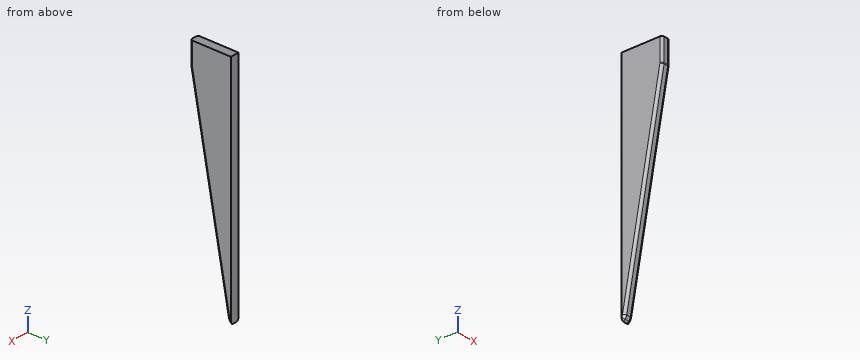
```python
from build123d import *

# Parameters (mm, degrees)
F1_DEPTH     = 19.05
F2_T1_DEPTH  = 453.2334559577
F2_T3_DEPTH  = 17.7217096423
F2_T5_DEPTH  = 62.3469086479
F2_T8_ANGLE  = 10.3758449201
F2_T10_ANGLE = 34.6241550799
F2_T12_ANGLE = 10.3758449201
F2_T14_ANGLE = 34.6241550799


# Not quite as in the source:
# - a fillet or chamfer that OpenCascade refuses, or shapes differently, is made with other operations: its cross-section is extruded or revolved along the edge and cut away or added


with BuildPart() as f1:
    # F0 (on Right) → F1 (new body)
    with BuildSketch(Plane.YZ):
        with BuildLine():
            Line((42.4285726043, -178.7500022879), (42.4285726043, 329.2499977121))
            Line((42.4285726043, 329.2499977121), (-46.4714273957, 329.2499977121))
            Line((-46.4714273957, 329.2499977121), (-46.4714273957, 279.6030890642))
            ThreePointArc((-46.4714273957, 279.6030890642), (-46.4194016068, 278.4547213725), (-46.2637504894, 277.3157623006))
            Line((-46.2637504894, 277.3157623006), (35.3656206904, -168.5061879892))
            ThreePointArc((35.3656206904, -168.5061879892), (36.6122005726, -172.1199848152), (38.877687663, -175.1991173466))
            Line((38.877687663, -175.1991173466), (42.4285726043, -178.7500022879))
        make_face()
    extrude(amount=F1_DEPTH)

    # F2: fillet of radius 5.08 on 2 edges, made by hand

    # F2_s2 → F2_t1 (cut)
    with BuildSketch(Plane(origin=(0, -50.6297547862, 276.5163530631), x_dir=(1, 0, 0), z_dir=(0, 0.1801044696, -0.9836474877))):
        with BuildLine():
            ThreePointArc((13.97, -4.4385863345), (17.5621024484, -5.9264838861), (19.05, -9.5185863345))
            Line((19.05, -9.5185863345), (19.05, -4.4385863345))
            Line((19.05, -4.4385863345), (13.97, -4.4385863345))
        make_face()
        with BuildLine():
            ThreePointArc((5.08, -4.4385863345), (1.4878975516, -5.9264838861), (0, -9.5185863345))
            Line((0, -9.5185863345), (0, -4.4385863345))
            Line((0, -4.4385863345), (5.08, -4.4385863345))
        make_face()
    extrude(amount=F2_T1_DEPTH, mode=Mode.SUBTRACT)

    # F2_s4 → F2_t3 (cut)
    with BuildSketch(Plane(origin=(0, 107.0384025048, -107.0384025048), x_dir=(1, 0, 0), z_dir=(0, 0.7071067812, -0.7071067812))):
        with BuildLine():
            ThreePointArc((5.08, 96.3938073503), (1.4878975516, 94.9059097987), (0, 91.3138073503))
            Line((0, 91.3138073503), (0, 96.3938073503))
            Line((0, 96.3938073503), (5.08, 96.3938073503))
        make_face()
        with BuildLine():
            ThreePointArc((13.97, 96.3938073503), (17.5621024484, 94.9059097987), (19.05, 91.3138073503))
            Line((19.05, 91.3138073503), (19.05, 96.3938073503))
            Line((19.05, 96.3938073503), (13.97, 96.3938073503))
        make_face()
    extrude(amount=F2_T3_DEPTH, mode=Mode.SUBTRACT)

    # F2_s6 → F2_t5 (cut)
    with BuildSketch(Plane.XY.offset(279.6030890642)):
        with BuildLine():
            ThreePointArc((5.08, -46.4714273957), (1.4878975516, -44.9835298442), (0, -41.3914273957))
            Line((0, -41.3914273957), (0, -46.4714273957))
            Line((0, -46.4714273957), (5.08, -46.4714273957))
        make_face()
        with BuildLine():
            ThreePointArc((13.97, -46.4714273957), (17.5621024484, -44.9835298442), (19.05, -41.3914273957))
            Line((19.05, -41.3914273957), (19.05, -46.4714273957))
            Line((19.05, -46.4714273957), (13.97, -46.4714273957))
        make_face()
    extrude(amount=F2_T5_DEPTH, mode=Mode.SUBTRACT)

    # F2_s7 → F2_t8 (revolve, cut)
    with BuildSketch(Plane.XY.offset(279.6030890642)):
        with BuildLine():
            ThreePointArc((5.08, -46.4714273957), (1.4878975516, -44.9835298442), (0, -41.3914273957))
            Line((0, -41.3914273957), (0, -46.4714273957))
            Line((0, -46.4714273957), (5.08, -46.4714273957))
        make_face()
    revolve(axis=Axis((0, -33.7714273957, 279.6030890642), (1, 0, 0)), revolution_arc=F2_T8_ANGLE, mode=Mode.SUBTRACT)

    # F2_s9 → F2_t10 (revolve, cut)
    with BuildSketch(Plane(origin=(0, 30.9996163936, -169.3055972266), x_dir=(1, 0, 0), z_dir=(0, -0.1801044696, 0.9836474877))):
        with BuildLine():
            ThreePointArc((5.08, 4.4385863345), (1.4878975516, 5.9264838861), (0, 9.5185863345))
            Line((0, 9.5185863345), (0, 4.4385863345))
            Line((0, 4.4385863345), (5.08, 4.4385863345))
        make_face()
    revolve(axis=Axis((0, 47.8579437841, -166.2188612255), (1, 0, 0)), revolution_arc=F2_T10_ANGLE, mode=Mode.SUBTRACT)

    # F2_s11 → F2_t12 (revolve, cut)
    with BuildSketch(Plane.XY.offset(279.6030890642)):
        with BuildLine():
            ThreePointArc((13.97, -46.4714273957), (17.5621024484, -44.9835298442), (19.05, -41.3914273957))
            Line((19.05, -41.3914273957), (19.05, -46.4714273957))
            Line((19.05, -46.4714273957), (13.97, -46.4714273957))
        make_face()
    revolve(axis=Axis((19.05, -33.7714273957, 279.6030890642), (1, 0, 0)), revolution_arc=F2_T12_ANGLE, mode=Mode.SUBTRACT)

    # F2_s13 → F2_t14 (revolve, cut)
    with BuildSketch(Plane(origin=(0, 30.9996163936, -169.3055972266), x_dir=(1, 0, 0), z_dir=(0, -0.1801044696, 0.9836474877))):
        with BuildLine():
            ThreePointArc((13.97, 4.4385863345), (17.5621024484, 5.9264838861), (19.05, 9.5185863345))
            Line((19.05, 9.5185863345), (19.05, 4.4385863345))
            Line((19.05, 4.4385863345), (13.97, 4.4385863345))
        make_face()
    revolve(axis=Axis((19.05, 47.8579437841, -166.2188612255), (1, 0, 0)), revolution_arc=F2_T14_ANGLE, mode=Mode.SUBTRACT)


solid = f1.part
```
CAD build for the part. Positions are in the model's coordinates, mm. Give positions to 0.01 mm unless a question says otherwise; leave off trailing zeros. Loops run counter-clockwise (first coordinate to the right, second up) from the corner with the lowest first, then second, coordinate; pieces in that order, holes last. Notation, with made-up numbers: (32, 58.25) - (50, 58.25) arc R27 ccw to (50, 96.25) - close; hole circle Ø3 at (47, 48). An arc over 180 degrees is marked (long way). Put each result on its own line as item: value.
Q1. Probe line 1 along Y through (x, z) = (15.25, 278.5); line 2 along Y through (x, z) = (2.5, -20); line 3 along X through (y, z) = (-12.5, 105). List the from-to ranges inside material, lowest first.
Filled in:
line 1: y = -46.26 to 42.43
line 2: y = 8.89 to 42.43
line 3: x = 0.91 to 18.14
Q2. Slice it at A-A (x = 10). Give the cut face in (y, z), plus the area to 3 significant figures.
Filled in:
outline: (-46.47, 279.6) arc R12.7 ccw to (-46.26, 277.32) - (35.37, -168.51) arc R12.7 ccw to (38.88, -175.2) - (42.43, -178.75) - (42.43, 329.25) - (-46.47, 329.25) - close
area: 26,000 mm²
Q3. Flat gauge pins, fed straight in: pin 1 (2 mm diameter, centred on x = 12.5, z = -99.5, fed in from -Y); pin 2 (3 mm diameter, centred on y = 24, z = -37.5, fed in from -X). Where does each tip first touch, or does it go through?
Filled in:
pin 1: stops at y = 22.55
pin 2: stops at x = 0
